from build123d import *

# Parameters (mm, degrees)
F0_R        = 13
F0_R_2      = 7
F1_DEPTH    = 10
F2_R        = 10
F2_R_2      = 7
F3_DEPTH    = 5.5
F4_W        = 13.5
F4_H        = 13.5
F5_DEPTH    = 10.001
F6_T1_DEPTH = 18.5160584479


# Not quite as in the source:
# - a fillet or chamfer that OpenCascade refuses, or shapes differently, is made with other operations: its cross-section is extruded or revolved along the edge and cut away or added


with BuildPart() as f1:
    # F0 (on Top) → F1 (new body)
    with BuildSketch(Plane.XY):
        Circle(F0_R)
        Circle(F0_R_2, mode=Mode.SUBTRACT)
    extrude(amount=F1_DEPTH)

    # F2 (on face) → F3 (cut)
    with BuildSketch(Plane.XY.offset(10)):
        Circle(F2_R)
        Circle(F2_R_2, mode=Mode.SUBTRACT)
    extrude(amount=-F3_DEPTH, mode=Mode.SUBTRACT)

    # F4 (on face) → F5 (cut, through all)
    with BuildSketch(Plane.XY.offset(10)):
        with Locations((-6.75, 0)):
            Rectangle(F4_W, F4_H)
    extrude(amount=-F5_DEPTH, mode=Mode.SUBTRACT)

    # F6: chamfer of 1.5 on 2 edges, made by hand

    # F6_s2 → F6_t1 (cut)
    with BuildSketch(Plane.XY.offset(-4.2580292239)):
        with BuildLine():
            Line((-10.1773648706, 8.1750152332), (-9.4664670488, 6.6959219319))
            Line((-9.4664670488, 6.6959219319), (-9.4664670488, 6.6659219319))
            ThreePointArc((-9.4664670488, 6.6659219319), (-10.2883550352, 6.72), (-11.1102430216, 6.72))
            Line((-11.1102430216, 6.72), (-11.135882044, 6.7655769231))
            ThreePointArc((-11.135882044, 6.7655769231), (-10.669011075, 7.4801806583), (-10.2007911166, 8.1937558574))
            Line((-10.2007911166, 8.1937558574), (-10.1773648706, 8.1750152332))
        make_face()
        with BuildLine():
            Line((-10.1773648706, -8.1750152332), (-9.4664670488, -6.6959219319))
            Line((-9.4664670488, -6.6959219319), (-9.4664670488, -6.6659219319))
            ThreePointArc((-9.4664670488, -6.6659219319), (-10.2883550352, -6.72), (-11.1102430216, -6.72))
            Line((-11.1102430216, -6.72), (-11.135882044, -6.7655769231))
            ThreePointArc((-11.135882044, -6.7655769231), (-10.669011075, -7.4801806583), (-10.2007911166, -8.1937558574))
            Line((-10.2007911166, -8.1937558574), (-10.1773648706, -8.1750152332))
        make_face()
    extrude(amount=F6_T1_DEPTH, mode=Mode.SUBTRACT)


solid = f1.part
Geometry: final body of the model. Coordinates: model frame, mm. A direction names the side the tool comes from. Give positions to 0.01 mm unless a question says otherwise; leave off trailing zeros. Order: outer loops, then holes, each group sorted by start corner. A loop starts at its lowest first (then second) coordinate and runs counter-clockwise, first axis right, second up. Notation, with made-up numbers: (-38, 32) -> (19, 32) arc R12 ccw to (19, 53) -> close; hole circle Ø8 at (77, 1.25). An arc over 180 degrees is marked (long way). Put each result on its own line as item: value.
Q1. Pin query (flat end, axial travel): pin 1 (2.5 mm diameter, centred on x = -6, z = 6, fed in from +Y); pin 2 (2 mm diameter, centred on y = -1.5, z = 3.5, fed in from -X); pin 3 (3 mm diameter, centred on y = -10, z = 5.5, fed in from -X); pin 4 (8 mm diameter, centred on x = 1.5, y = -0.5, fed in from -Z). Return the tip coordinate at first contact, or that it passes through.
Here are the results:
pin 1: stops at y = 12.1
pin 2: stops at x = 6.54
pin 3: stops at x = -9.84
pin 4: passes through
Q2. Section D-D, the plane x = 5.75. Return loops of the section in (y, z).
Here are the results:
outline: (-11.66, 0) -> (-3.99, 0) -> (-3.99, 4.5) -> (-8.18, 4.5) -> (-8.18, 10) -> (-11.66, 10) -> close; (3.99, 0) -> (11.66, 0) -> (11.66, 10) -> (8.18, 10) -> (8.18, 4.5) -> (3.99, 4.5) -> close
Q3. Section B-B, the plane z = 8.25. Return loops of the section in (x, y).
Here are the results:
outline: (-10.15, -8.12) arc R13 ccw (long way) to (-10.15, 8.12) -> (-9.49, 6.75) -> (-7.38, 6.75) arc R10 cw (long way) to (-7.38, -6.75) -> (-9.49, -6.75) -> close
Q4. Section A-A, the plane x = 0. Return loops of the section in (y, z).
Here are the results:
outline: (-13, 0) -> (-7, 0) -> (-7, 4.5) -> (-10, 4.5) -> (-10, 10) -> (-13, 10) -> close; (7, 0) -> (13, 0) -> (13, 10) -> (10, 10) -> (10, 4.5) -> (7, 4.5) -> close
Q5. Section C-C, the plane y = -0.75. Return loops of the section in (x, z).
Here are the results:
outline: (6.96, 0) -> (12.98, 0) -> (12.98, 10) -> (9.97, 10) -> (9.97, 4.5) -> (6.96, 4.5) -> close
Q6. Material intervals for L1, parallel to Y at x = 0, z = 3.35; L2, parallel to Y at x = 0, z = 6.65; L3, parallel to X at y = 0, z = 6.4, sorted ascending.
Here are the results:
L1: y = -13 to -7, 7 to 13
L2: y = -13 to -10, 10 to 13
L3: x = 10 to 13
Q7. Reachability of faces 1 (the face through (7, 0, 2)), 2 (the face through (-9.83, 7.45, 4.93)), 3 (the face through (7, 2, 4.5)) from +Z, -Z, +X, -X, +Y, -Y: full face, straight path, thin tool, end or side. Return the list, or none.
Here are the results:
face 1: +Z, -Z
face 2: +Z, -Z, -X
face 3: +Z
